Read the model definition and answer for the solid it produces. Units are mm, in the model's axes. A direction names the side the tool comes from. Give positions to 0.01 mm unless a question says otherwise; leave off trailing zeros. Write each loop counter-clockwise with the first axis right and the second up, starting at its lowest first coordinate (ties: lowest second). Pieces come first, ordered by that corner, then holes. Notation, with made-up numbers: (-21.75, 7.25) - (22.25, 7.25) arc R27 cw to (22.25, 45.25) - close; hole circle Ø6 at (80, 12.5). An arc over 180 degrees is marked (long way). Use CSV: the item, a comma, the result in double quotes. Start each with the question number.
from build123d import *

# Parameters (mm, degrees)
BOSS_EXTRUDE1_REACH                  = 105.503
BOSS_EXTRUDE1_END_RADIUS             = 45.72
BOSS_EXTRUDE1_DIRECTION_2_REACH      = 105.503
BOSS_EXTRUDE1_DIRECTION_2_END_RADIUS = 45.72
EXTRUDE_THIN1_START                  = -2.54
SKETCH3_R                            = 45.72
SKETCH3_R_2                          = 26.67
EXTRUDE_THIN1_DEPTH                  = 2.54


with BuildPart() as part:
    # Sketch1 → Revolve1 (revolve)
    with BuildSketch(Plane(origin=(0, 0, 0), x_dir=(0, 0, -1), z_dir=(1, 0, 0)), mode=Mode.PRIVATE) as revolve1_sk:
        Polygon((-49.53, 0), (-49.53, -76.2), (-45.72, -76.2), (-45.72, -10.104637547), (-41.402, -0.844656665), (-41.402, 10.16), (-45.212, 10.16), (-45.212, 0), align=None)
    revolve(revolve1_sk.sketch.rotate(Axis((0, 0, 0), (0, 1, 0)), 180), axis=Axis((0, 0, 0), (0, 1, 0)))

    # Boss-Extrude1: up to this cylinder (the profile starts inside it)
    boss_extrude1_end = Plane(origin=(0, -73.102853, 0), z_dir=(0, -1, 0)) * Cylinder(BOSS_EXTRUDE1_END_RADIUS, 303.446, mode=Mode.PRIVATE)
    # Sketch2 → Boss-Extrude1 (add, up to the surface)
    with BuildSketch(Plane(origin=(0, 0, 0), x_dir=(0, 0, -1), z_dir=(1, 0, 0)), mode=Mode.PRIVATE) as boss_extrude1_sk1:
        with BuildLine():
            Line((4.445, -73.66), (4.445, -76.2))
            Line((4.445, -76.2), (-4.445, -76.2))
            Line((-4.445, -76.2), (-4.445, -73.66))
            ThreePointArc((-4.445, -73.66), (0, -69.215), (4.445, -73.66))
        make_face()
    boss_extrude1_tool1 = extrude(boss_extrude1_sk1.sketch, amount=BOSS_EXTRUDE1_REACH, mode=Mode.PRIVATE) & boss_extrude1_end
    add(boss_extrude1_tool1.solids().sort_by_distance((0, -73.102853, 0))[0])

    # Boss-Extrude1 direction 2: up to this cylinder (the profile starts inside it)
    boss_extrude1_direction_2_end = Plane(origin=(0, -73.102853, 0), z_dir=(0, -1, 0)) * Cylinder(BOSS_EXTRUDE1_DIRECTION_2_END_RADIUS, 303.446, mode=Mode.PRIVATE)
    # Sketch2 → Boss-Extrude1 direction 2 (add, up to the surface)
    with BuildSketch(Plane(origin=(0, 0, 0), x_dir=(0, 0, -1), z_dir=(1, 0, 0)), mode=Mode.PRIVATE) as boss_extrude1_direction_2_sk1:
        with BuildLine():
            Line((4.445, -73.66), (4.445, -76.2))
            Line((4.445, -76.2), (-4.445, -76.2))
            Line((-4.445, -76.2), (-4.445, -73.66))
            ThreePointArc((-4.445, -73.66), (0, -69.215), (4.445, -73.66))
        make_face()
    boss_extrude1_direction_2_tool1 = extrude(boss_extrude1_direction_2_sk1.sketch, amount=-BOSS_EXTRUDE1_DIRECTION_2_REACH, mode=Mode.PRIVATE) & boss_extrude1_direction_2_end
    add(boss_extrude1_direction_2_tool1.solids().sort_by_distance((0, -73.102853, 0))[0])

    # Sketch3 → Extrude-Thin1 (add)
    with BuildSketch(Plane.XZ.offset(76.2).offset(EXTRUDE_THIN1_START)):
        Circle(SKETCH3_R)
        Circle(SKETCH3_R_2, mode=Mode.SUBTRACT)
    extrude(amount=EXTRUDE_THIN1_DEPTH)


solid = part.part
(1) The part is cut by section A-A on x = 0. Write down the section's boundary in (y, z) (3 decimals).
(2) Consider probe 1 along X at (y, z) = (-39, 0); probe 2 along X at (y, z) = (4, 0); probe 3 along Z at (x, y) = (-39.5, -72). Determine where each line is inside the solid, lowest interval first.
(3) The part is cut by section B-B on z = 0. Write down the section's boundary in (x, y) (3 decimals), plus the area to 3 significant figures.
(4) The part is cut by section C-C on y = -57. Write down the section's boundary in (x, z), plus the area to 3 significant figures.
(5) For a pull along Y with two mould halves and no side action, classify faces 5 (the face through (20, 10.16, 37)), 6 (the face through (-1, -73.66, 30)), 7 (the face through (40.417, 4.735, 8.975)) as pulls with the +Y half, pulls with the -Y half, needs draft (parallel to the pull), parting line crosses it, or undercut.
(6) Given P1, Ø3, axis at y = -15, z = 22, coming from the +X side; P2, Ø1.5, axis at x = 20, y = -56, coming from the -Z side; P3, Ø10, axis at x = 25.5, z = -8.5, coming from the +Y side, each flat-ended and moving along its own axis, determine where each tip first touches the part or whether it passes through.
(7) The part is cut by section D-D on y = 3. Write down the section's boundary in (x, z), plus the area to 3 significant figures.
(8) Which of the six approach directions +Z, -Z, +X, -X, +Y, -Y give full straight-line access (tool end or side, diameter ignored) to faces 1 (the face through (1, -76.2, -1)), 2 (the face through (17.511, -41.437, -42.234)), 3 (the face through (0, -75, -4.445)), 4 (the face through (44.137, 5.009, 9.801))?
Reported:
1,outline,"(-76.2, -49.53) - (0, -49.53) - (0, -45.212) - (10.16, -45.212) - (10.16, -41.402) - (-0.845, -41.402) - (-10.105, -45.72) - (-73.66, -45.72) - (-73.66, -26.67) - (-76.2, -26.67) - close; (-76.2, -4.445) - (-73.66, -4.445) arc R4.445 ccw to (-73.66, 4.445) - (-76.2, 4.445) - close; (-76.2, 26.67) - (-73.66, 26.67) - (-73.66, 45.72) - (-10.105, 45.72) - (-0.845, 41.402) - (10.16, 41.402) - (10.16, 45.212) - (0, 45.212) - (0, 49.53) - (-76.2, 49.53) - close"
2,probe 1,"-49.53 to -45.72, 45.72 to 49.53"
2,probe 2,"-45.21 to -41.4, 41.4 to 45.21"
2,probe 3,"-29.88 to -23.02, -4.12 to 4.12, 23.02 to 29.88"
3,outline,"(-49.53, -76.2) - (49.53, -76.2) - (49.53, 0) - (45.212, 0) - (45.212, 10.16) - (41.402, 10.16) - (41.402, -0.845) - (45.72, -10.105) - (45.72, -69.215) - (-45.72, -69.215) - (-45.72, -10.105) - (-41.402, -0.845) - (-41.402, 10.16) - (-45.212, 10.16) - (-45.212, 0) - (-49.53, 0) - close"
3,area,"1,340 mm²"
4,outline,"circle Ø99.06 at (0, 0); hole circle Ø91.44 at (0, 0)"
4,area,"1,140 mm²"
5,face 5,"pulls with the +Y half"
5,face 6,"undercut"
5,face 7,"needs draft"
6,P1,"x = 45.09"
6,P2,"z = -45.64"
6,P3,"y = -70.92"
7,outline,"circle Ø90.42 at (0, 0); hole circle Ø82.8 at (0, 0)"
7,area,"1,040 mm²"
8,face 1,"+Z, -Z, +X, -X, -Y"
8,face 2,"none"
8,face 3,"+Y, -Y"
8,face 4,"+Y"
